Part model, mm, in its own coordinate system. A direction names the side the tool comes from. Coordinates: 2 decimals unless noted, no trailing zeros. Order: outer loops, then holes, each group sorted by start corner. A loop starts at its lowest first (then second) coordinate and runs counter-clockwise, first axis right, second up. Notation, with made-up numbers: (-27, 25) - (7, 25) arc R18 ccw to (7, 60) - close; hole circle Ø1 at (-31.75, 16.25). An arc over 180 degrees is marked (long way). Use a Markdown table: item, result. Add a question column.
1) Wall check: L1, parallel to Y at x = -1.35, z = 17; L2, parallel to Z at x = 14, y = 1; L3, parallel to Y at x = 0.95, z = 17. Give the ranges that are in metal, low to high. Write a range as [from, to].
2) Saw through at A-A on x = 14. List the corners of the cut face in (y, z), then the cut area to 3 significant figures.
3) Saw through at D-D on z = 8.75. List the corners of the cut face in (x, y).
4) Tool access for faces 1 (the face through (4, 18, 10)), 2 (the face through (-1, 28, 19)), 3 (the face through (3.5, 8.6, 0)): list every direction of +Z, -Z, +X, -X, +Y, -Y with a clear straight run to the whole face (end or side of a thin tool).
5) Two-plate mould, pull along Z, no slides. Class faces 4 (the face through (2.03, 28.4, 0.57)), 5 (the face through (13.772, 2.028, 14.265)), 6 (the face through (12, 4, 10)): +Z half, -Z half, draft (parallel to the pull), parting line (faces both ways), or undercut.
6) Drop flat-ended pins along their axis: P1, Ø6.5, axis at x = 13.5, z = 9, coming from the +Y side; P2, Ø12, axis at y = 15.5, z = 14.5, coming from the +X side; P3, Ø6, axis at y = 22, z = 2.5, coming from the -X side. Give the stop position or say it passes through.
7) Saw through at C-C on y = 26.5. List the corners of the cut face in (x, z).
8) Saw through at B-B on y = 2.75. List the corners of the cut face in (x, z), then the cut area to 3 significant figures.
```python
from build123d import *

# Parameters (mm, degrees)
BOSS_EXTRUDE1_DEPTH = 20
SKETCH2_R           = 1.5
CUT_EXTRUDE1_DEPTH  = 20
SKETCH3_R           = 1.75
CUT_EXTRUDE2_DEPTH  = 5
FILLET1_R           = 2
BOSS_EXTRUDE2_START = -4
SKETCH4_R           = 2.5
SKETCH4_R_2         = 1.5
BOSS_EXTRUDE2_DEPTH = 2


with BuildPart() as part:
    # Sketch1 → Boss-Extrude1 (new body)
    with BuildSketch(Plane.XY):
        Polygon((0, 0), (0, 29), (4, 29), (4, 4), (19, 4), (19, 0), align=None)
    extrude(amount=BOSS_EXTRUDE1_DEPTH)

    # Sketch2 → Cut-Extrude1 (cut, through all)
    with BuildSketch(Plane.ZY):
        with Locations((17, 26.5)):
            Circle(SKETCH2_R)
        with Locations((17, 11.5)):
            Circle(SKETCH2_R)
    extrude(amount=-CUT_EXTRUDE1_DEPTH, mode=Mode.SUBTRACT)

    # Sketch3 → Cut-Extrude2 (cut, through all)
    with BuildSketch(Plane(origin=(0, 4, 0), x_dir=(1, 0, 0), z_dir=(0, 1, 0))):
        with Locations((14, -4)):
            Circle(SKETCH3_R)
        with Locations((14, -16)):
            Circle(SKETCH3_R)
    extrude(amount=-CUT_EXTRUDE2_DEPTH, mode=Mode.SUBTRACT)

    # Fillet1
    fillet1_edges = [part.edges().sort_by_distance(p)[0] for p in [
        (4, 4, 10),
        (2, 29, 20),
        (2, 29, 0),
        (19, 2, 0),
        (19, 2, 20),
    ]]
    fillet(fillet1_edges, radius=FILLET1_R)

    # Sketch4 → Boss-Extrude2 (add)
    with BuildSketch(Plane(origin=(4, 0, 0), x_dir=(0, 0, -1), z_dir=(1, 0, 0)).offset(BOSS_EXTRUDE2_START)):
        with Locations((-17, 26.5)):
            Circle(SKETCH4_R)
        with Locations((-17, 26.5)):
            Circle(SKETCH4_R_2, mode=Mode.SUBTRACT)
        with Locations((-17, 11.5)):
            Circle(SKETCH4_R)
        with Locations((-17, 11.5)):
            Circle(SKETCH4_R_2, mode=Mode.SUBTRACT)
    extrude(amount=-BOSS_EXTRUDE2_DEPTH)


solid = part.part
```
Results are:
| question | item | result |
|---|---|---|
| 1 | L1 | [9, 10], [13, 14], [24, 25], [28, 29] |
| 1 | L2 | [0, 2.25], [5.75, 14.25], [17.75, 20] |
| 1 | L3 | [0, 10], [13, 25], [28, 29] |
| 2 | outline | (0, 0) - (4, 0) - (4, 2.25) - (0, 2.25) - close; (0, 5.75) - (4, 5.75) - (4, 14.25) - (0, 14.25) - close; (0, 17.75) - (4, 17.75) - (4, 20) - (0, 20) - close |
| 2 | area | 52.0 mm2 |
| 3 | outline | (0, 0) - (19, 0) - (19, 4) - (6, 4) arc R2 cw to (4, 6) - (4, 29) - (0, 29) - close |
| 4 | face 1 | +Z, -Z, +X, +Y |
| 4 | face 2 | -X |
| 4 | face 3 | -Z, +X, -X, +Y, -Y |
| 5 | face 4 | -Z half |
| 5 | face 5 | undercut |
| 5 | face 6 | draft |
| 6 | P1 | y = 4 |
| 6 | P2 | x = 4 |
| 6 | P3 | x = 0 |
| 7 | outline | (-2, 14.5) - (0, 14.5) - (0, 0) - (4, 0) - (4, 15.5) - (-2, 15.5) - close; (-2, 18.5) - (4, 18.5) - (4, 20) - (0, 20) - (0, 19.5) - (-2, 19.5) - close |
| 8 | outline | (0, 0) - (17, 0) arc R2 ccw to (19, 2) - (19, 18) arc R2 ccw to (17, 20) - (0, 20) - close; hole circle Ø3.5 at (14, 4); hole circle Ø3.5 at (14, 16) |
| 8 | area | 359 mm2 |
